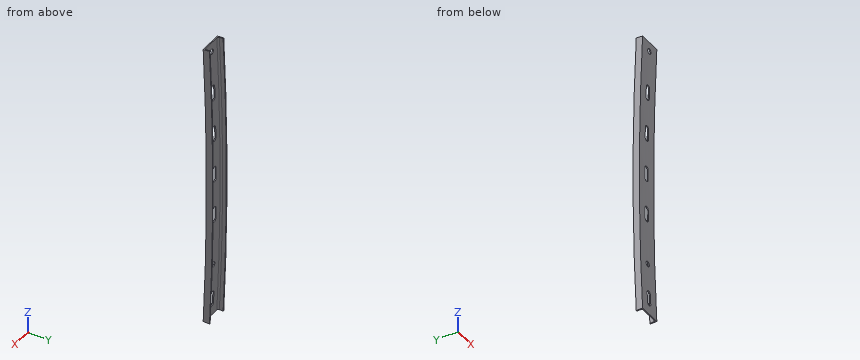
```python
from build123d import *

# Parameters (mm, degrees)
VARIOUS_MOUNTING_POINTS_DEPTH      = 302.472328172
VARIOUS_MOUNTING_POINTS_DEPTH_BACK = 302.472328172
SKETCH4_R                          = 5


with BuildPart() as part:
    # Sweep1: sweep along a path in Sketch3
    with BuildLine(Plane(origin=(0, 0, 0), x_dir=(0, 0, -1), z_dir=(1, 0, 0))) as sweep1_path:
        ThreePointArc((-240, -6), (30, 0.074962051), (300, -6))
    # Sketch1 → Sweep1 (sweep)
    with BuildSketch(Plane.XY):
        with BuildLine():
            Line((-17, 0), (17, 0))
            ThreePointArc((17, 0), (19.121320344, 0.878679656), (20, 3))
            Line((20, 3), (20, 10))
            Line((20, 10), (22, 10))
            Line((22, 10), (22, -2))
            Line((22, -2), (-22, -2))
            Line((-22, -2), (-22, 10))
            Line((-22, 10), (-20, 10))
            Line((-20, 10), (-20, 3))
            ThreePointArc((-20, 3), (-19.121320344, 0.878679656), (-17, 0))
        make_face()
    sweep(path=sweep1_path.line)

    # Sketch4 → Various mounting points (cut, two sides: drawn at the far end of the back side and taken through both)
    with BuildSketch(Plane(origin=(0, 0, 0), x_dir=(1, 0, 0), z_dir=(0, 1, 0)).offset(-VARIOUS_MOUNTING_POINTS_DEPTH_BACK)):
        with Locations(Location((0, 197.900062461, 0), (0, 0, 270))):
            Circle(SKETCH4_R)
        with Locations(Location((0, -223.099937539, 0), (0, 0, 270))):
            Circle(SKETCH4_R)
        with BuildLine():
            Line((-5, 256.900062461), (-5, 276.900062461))
            ThreePointArc((-5, 276.900062461), (0, 281.900062461), (5, 276.900062461))
            Line((5, 276.900062461), (5, 256.900062461))
            ThreePointArc((5, 256.900062461), (0, 251.900062461), (-5, 256.900062461))
        make_face()
        with BuildLine():
            Line((-5, 87.900062461), (-5, 107.900062461))
            ThreePointArc((-5, 107.900062461), (0, 112.900062461), (5, 107.900062461))
            Line((5, 107.900062461), (5, 87.900062461))
            ThreePointArc((5, 87.900062461), (0, 82.900062461), (-5, 87.900062461))
        make_face()
        with BuildLine():
            Line((-5, 7.900062461), (-5, 27.900062461))
            ThreePointArc((-5, 27.900062461), (0, 32.900062461), (5, 27.900062461))
            Line((5, 27.900062461), (5, 7.900062461))
            ThreePointArc((5, 7.900062461), (0, 2.900062461), (-5, 7.900062461))
        make_face()
        with BuildLine():
            Line((-5, -72.099937539), (-5, -52.099937539))
            ThreePointArc((-5, -52.099937539), (0, -47.099937539), (5, -52.099937539))
            Line((5, -52.099937539), (5, -72.099937539))
            ThreePointArc((5, -72.099937539), (0, -77.099937539), (-5, -72.099937539))
        make_face()
        with BuildLine():
            Line((-5, -152.099937539), (-5, -132.099937539))
            ThreePointArc((-5, -132.099937539), (0, -127.099937539), (5, -132.099937539))
            Line((5, -132.099937539), (5, -152.099937539))
            ThreePointArc((5, -152.099937539), (0, -157.099937539), (-5, -152.099937539))
        make_face()
    extrude(amount=VARIOUS_MOUNTING_POINTS_DEPTH + VARIOUS_MOUNTING_POINTS_DEPTH_BACK, mode=Mode.SUBTRACT)


solid = part.part
```
Check sheet for the modelled part. Datum: model origin and axes. Units: mm. Round coordinates to 2 decimals unless told otherwise and drop trailing zeros. Answer as a JSON object with one key per item and string values.
1. Section check A-A (x = 0). State how many separate pieces and enclosed holes the cut face has, plus the area to 3 significant figures.
Reply:
{"separate pieces": "8", "enclosed holes": "0", "area": "740 mm²"}
2. Gauge pin test, flat ends, axial feed: P1, Ø6, axis at x = -0.5, y = -4.5, coming from the +Z side; P2, Ø11.5, axis at x = 0, z = -197.9, coming from the +Y side; P3, Ø1, axis at x = -1, y = -6, coming from the -Z side; P4, Ø4, axis at y = -4.5, z = 7, coming from the +X side. Record the tip position at first contact, or that the pin passes through.
Reply:
{"P1": "stops at z = 240", "P2": "stops at y = -2.12", "P3": "stops at z = -300", "P4": "passes through"}
3. Scan lines: line 1 (X direction, y = 8.75, z = -143.5); line 2 (X direction, y = -1.75, z = -24); line 3 (Y direction, x = 4, z = 19.5). Record each from-to range of solid material in increasing order.
Reply:
{"line 1": "x = -22 to -20, 20 to 22", "line 2": "x = -22 to -5, 5 to 22", "line 3": "y = -2.13 to -0.13"}
